For this review, take the finished solid that the model builds, in its own axes (mm). Face numbers are marked on the shaded views. A direction names the side the tool comes from. Round coordinates to 2 decimals unless told otherwise and drop trailing zeros. Loops run counter-clockwise (first coordinate to the right, second up) from the corner with the lowest first, then second, coordinate; pieces in that order, holes last. Notation, with made-up numbers: M -15.5,42.25 L 26.5,42.25 A27 ccw 26.5,64.25 Z; hole C 22.5,76.25 d11. An arc over 180 degrees is marked long. One line per question, with ' | ' between items. Start each with the question number.
1) For the marked faces 5, 6, 7, 8 and 9, list the 3-axis set-ups (+Z, -Z, +X, -X, +Y, -Y) from which the entire face can be reached by the end or side of a thin tool; tool diameter is ignored.
2) We need section B-B (z = 1.95). State how many separate pieces and enclosed holes the cut face has, and give its area (3 significant figures).
3) Mouldability with a two-part tool opening along X and no side actions: class the marked faces 1, 2, 3 and 4 as pulls with the +X half, pulls with the -X half, needs draft (parallel to the pull), parting line crosses it, or undercut.
4) For probe 1 along Y at (x, z) = (0, 4.65); probe 2 along X at (y, z) = (0.75, 3.45); probe 3 along X at (y, z) = (-2.25, 0.6), list the stretches that pass through material, from the lowest coordinate up. Write a range as from..to.
5) For pin 1 Ø1 at (x, z) = (-25, 3) entering from -Y; pin 2 Ø3 at (x, z) = (-7.5, 1) entering from +Y; pin 3 Ø10 at (x, y) = (3.5, 1.5) entering from +Z, all flat-tipped, find the tip position at first contact; note any pin that passes through.
6) We need section A-A (z = 4.65). Give the boundary of the cut face in (x, y).
7) We need section C-C (x = 21). Give the boundary of the cut face in (y, z).
```python
from build123d import *

# Parameters (mm, degrees)
F0_R     = 2.45
F1_DEPTH = 6
F2_R     = 10
F3_DEPTH = 3
F4_W     = 2.8
F4_H     = 2.8
F5_DEPTH = 3.001


with BuildPart() as f1:
    # F0 (on Top) → F1 (new body)
    with BuildSketch(Plane.XY):
        with BuildLine():
            ThreePointArc((10.246951, -8), (12.292485, -4.230227), (13, 0))
            ThreePointArc((13, 0), (12.292485, 4.230227), (10.246951, 8))
            ThreePointArc((10.246951, 8), (0, 13), (-10.246951, 8))
            ThreePointArc((-10.246951, 8), (-13, 0), (-10.246951, -8))
            ThreePointArc((-10.246951, -8), (0, -13), (10.246951, -8))
        make_face()
        with BuildLine():
            ThreePointArc((10.246951, 8), (12.292485, 4.230227), (13, 0))
            ThreePointArc((13, 0), (12.292485, -4.230227), (10.246951, -8))
            Line((10.246951, -8), (32.370236, -8))
            Line((32.370236, -8), (32.370236, 8))
            Line((32.370236, 8), (10.246951, 8))
        make_face()
        with Locations((24.920236, 0)):
            Circle(F0_R, mode=Mode.SUBTRACT)
        with BuildLine():
            ThreePointArc((-10.246951, -8), (-13, 0), (-10.246951, 8))
            Line((-10.246951, 8), (-31.858318, 8))
            Line((-31.858318, 8), (-31.858318, -8))
            Line((-31.858318, -8), (-10.246951, -8))
        make_face()
        with Locations((-24.408318, 0)):
            Circle(F0_R, mode=Mode.SUBTRACT)
    extrude(amount=F1_DEPTH)

    # F2 (on face) → F3 (cut)
    with BuildSketch(Plane.XY.offset(6)):
        Circle(F2_R)
    extrude(amount=-F3_DEPTH, mode=Mode.SUBTRACT)

    # F4 (on face) → F5 (cut, through all)
    with BuildSketch(Plane.XY.offset(3)):
        with Locations((-7.84869, -0.110486)):
            Rectangle(F4_W, F4_H)
        Polygon((-4.609375, -4.756964), (-6.123169, -2.401454), (-8.478679, -3.915248), (-6.964885, -6.270758), align=None)
        Polygon((-1.306867, -6.493666), (-3.853836, -5.330504), (-5.016998, -7.877474), (-2.470029, -9.040636), align=None)
        Polygon((2.410312, -6.169202), (-0.361188, -6.567683), (0.037294, -9.339184), (2.808794, -8.940702), align=None)
        Polygon((5.361984, -3.886587), (3.245885, -5.720197), (5.079495, -7.836296), (7.195594, -6.002685), align=None)
        Polygon((6.611013, -0.370534), (5.822162, -3.057115), (8.508742, -3.845966), (9.297593, -1.159386), align=None)
        Polygon((5.760842, 3.262633), (6.549693, 0.576053), (9.236273, 1.364904), (8.447422, 4.051484), align=None)
        Polygon((3.081393, 5.859411), (5.197492, 4.025801), (7.031102, 6.141899), (4.915004, 7.975509), align=None)
        Polygon((-0.576626, 6.59534), (2.194874, 6.196858), (2.593356, 8.968358), (-0.178144, 9.36684), align=None)
        Polygon((-4.051821, 5.236769), (-1.504851, 6.399931), (-2.668013, 8.9469), (-5.214983, 7.783738), align=None)
        Polygon((-6.240842, 2.215033), (-4.727048, 4.570543), (-7.082557, 6.084338), (-8.596352, 3.728828), align=None)
    extrude(amount=-F5_DEPTH, mode=Mode.SUBTRACT)


solid = f1.part
```
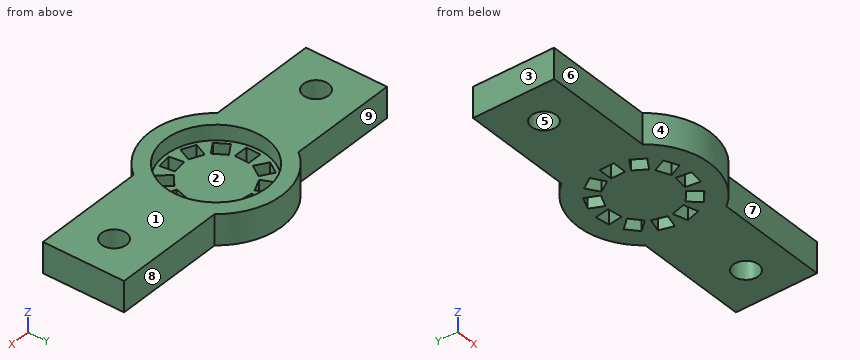
Answers below:
1) face 5: +Z, -Z | face 6: +Z, -Z, -X, -Y | face 7: +Z, -Z, +X, -Y | face 8: +Z, -Z, +X, +Y | face 9: +Z, -Z, -X, +Y
2) separate pieces: 1 | enclosed holes: 13 | area: 1,050 mm^2
3) face 1: needs draft | face 2: undercut | face 3: pulls with the -X half | face 4: parting line crosses it
4) probe 1: -13..-10, 10..13 | probe 2: -31.86..-26.74, -22.08..-9.97, 9.97..22.59, 27.25..32.37 | probe 3: -31.86..-25.38, -23.44..6.06, 8.98..23.95, 25.89..32.37
5) pin 1: y = -8 | pin 2: y = 11.53 | pin 3: z = 3
6) outline: M -31.86,-8 L -10.25,-8 A13 ccw 10.25,-8 L 32.37,-8 L 32.37,8 L 10.25,8 A13 ccw -10.25,8 L -31.86,8 Z; hole C -24.41,0 d4.9; hole C 0,0 d20; hole C 24.92,0 d4.9
7) outline: M -8,0 L 8,0 L 8,6 L -8,6 Z
